```python
from build123d import *

# Parameters (mm, degrees)
SKETCH_1_R               = 22.5
EXTRUDE_1_DEPTH          = 9.5
SKETCH_2_R               = 15
EXTRUDE_2_DEPTH          = 5
SKETCH_3_R               = 1.5
CUT_EXTRUDE_1_DEPTH      = 5
SKETCH_5_R               = 1.5
CUT_EXTRUDE_2_DEPTH      = 34.207679835
CUT_EXTRUDE_6_DEPTH      = 3
PATTERN_CIRCULAR_1_COUNT = 12


with BuildPart() as part:
    # 草图1 → 凸台-拉伸1 (new body)
    with BuildSketch(Plane.XY):
        Circle(SKETCH_1_R)
    extrude(amount=EXTRUDE_1_DEPTH)

    # 草图2 → 凸台-拉伸2 (add)
    with BuildSketch(Plane.XY.offset(9.5)):
        Circle(SKETCH_2_R)
    extrude(amount=EXTRUDE_2_DEPTH)

    # 草图3 → 切除-拉伸1 (cut)
    with BuildSketch(Plane.XY.offset(9.5)):
        with Locations((0, 18.5)):
            Circle(SKETCH_3_R)
    cut_extrude_1 = extrude(amount=-CUT_EXTRUDE_1_DEPTH, mode=Mode.SUBTRACT)

    # 草图5 → 切除-拉伸2 (cut, through all)
    with BuildSketch(Plane.XY.offset(9.5)):
        with Locations((0, 18.5)):
            Circle(SKETCH_5_R)
    cut_extrude_2 = extrude(amount=-CUT_EXTRUDE_2_DEPTH, mode=Mode.SUBTRACT)

    # 草图9 → 切除-拉伸6 (cut)
    with BuildSketch(Plane(origin=(0, 0, 0), x_dir=(-1, 0, 0), z_dir=(0, 0, -1))):
        Polygon((1.204492644, 21.438116881), (-1.942237536, 21.012179669), (-3.14673018, 18.074062788), (-1.204492644, 15.561883119), (1.942237536, 15.987820331), (3.14673018, 18.925937212), align=None)
    cut_extrude_6 = extrude(amount=-CUT_EXTRUDE_6_DEPTH, mode=Mode.SUBTRACT)

    # 阵列(圆周)1: 切除-拉伸1, 切除-拉伸2, 切除-拉伸6 ×12 about axis
    pattern_circular_1_axis = Axis((0, 0, 0), (0, 0, 1))
    add([cut_extrude_1.rotate(pattern_circular_1_axis, i * 360 / PATTERN_CIRCULAR_1_COUNT) for i in range(1, PATTERN_CIRCULAR_1_COUNT)], mode=Mode.SUBTRACT)
    add([cut_extrude_2.rotate(pattern_circular_1_axis, i * 360 / PATTERN_CIRCULAR_1_COUNT) for i in range(1, PATTERN_CIRCULAR_1_COUNT)], mode=Mode.SUBTRACT)
    add([cut_extrude_6.rotate(pattern_circular_1_axis, i * 360 / PATTERN_CIRCULAR_1_COUNT) for i in range(1, PATTERN_CIRCULAR_1_COUNT)], mode=Mode.SUBTRACT)


solid = part.part
```
Could you check a few things on this model? Use its own coordinates, in mm. A direction names the side the tool comes from. Give positions to 0.01 mm unless a question says otherwise; leave off trailing zeros. Order: outer loops, then holes, each group sorted by start corner. A loop starts at its lowest first (then second) coordinate and runs counter-clockwise, first axis right, second up.
Q1. Suppose I cut it at C-C, the plane z = 4.75. Count the separate pieces of the cut face and the enclosed holes in it, and give its area (3 significant figures).
Q2. Suppose I cut it at D-D, the plane y = 5.5. Write out the boundary of the cut face in (x, z).
Q3. Suppose I cut it at A-A, the plane y = 0. Write out the boundary of the cut face in (x, z), and give its area (3 significant figures).
Q4. Suppose I cut it at B-B, the plane x = 4.5. Write out the boundary of the cut face in (y, z), and give its area (3 significant figures).
Q5. We'd pull the mould along Y, two halves only. Please class faces 1 (the flat face through (8.186, -13.485, 1.479)), 2 (the cylindrical face through (10.382, -19.961, 4.684)): +Y half, -Y half, draft (parallel to the pull), parting line (faces both ways), or undercut.
Q6. If I drill on line 1 along Y through (x, z) = (0, 7.75); line 2 along X through (y, z) = (16, 8.25); line 3 along Z through (x, y) = (-17, -14), over which ranges is the centre line in solid material (lowest first)?
Q7. I'm going to push flat-ended pins straight in: P1, Ø2.5, axis at x = 18.5, y = 0, coming from the +Z side; P2, Ø3, axis at x = 16, y = 10, coming from the -Z side; P3, Ø1, axis at x = 3, z = 1.5, coming from the +Y side; P4, Ø5, axis at x = -16.02, y = -9.25, coming from the +Z side. Where does each tip first touch, or does it pass through?
Q8. For faces 3 (the flat face through (-16.836, 2.189, 1.479)), 4 (the cylindrical face through (9.825, -14.636, 6.296)), which set-ups out of +Z, -Z, +X, -X, +Y, -Y let a thin tool reach every point of the face, with its end or its side?
Solution:
1. separate pieces: 1
1. enclosed holes: 12
1. area: 1,510 mm2
2. outline: (-21.82, 0) - (21.82, 0) - (21.82, 9.5) - (13.96, 9.5) - (13.96, 14.5) - (-13.96, 14.5) - (-13.96, 9.5) - (-21.82, 9.5) - close
3. outline: (-22.5, 0) - (-21.28, 0) - (-21.28, 3) - (-20, 3) - (-20, 9.5) - (-22.5, 9.5) - close; (-17, 3) - (-15.72, 3) - (-15.72, 0) - (15.72, 0) - (15.72, 3) - (17, 3) - (17, 9.5) - (15, 9.5) - (15, 14.5) - (-15, 14.5) - (-15, 9.5) - (-17, 9.5) - close; (20, 3) - (21.28, 3) - (21.28, 0) - (22.5, 0) - (22.5, 9.5) - (20, 9.5) - close
3. area: 505 mm2
4. outline: (-22.05, 0) - (22.05, 0) - (22.05, 9.5) - (14.31, 9.5) - (14.31, 14.5) - (-14.31, 14.5) - (-14.31, 9.5) - (-22.05, 9.5) - close
4. area: 562 mm2
5. face 1: undercut
5. face 2: parting line
6. line 1: y = -22.5 to -20, -17 to 17, 20 to 22.5
6. line 2: x = -15.82 to -10.75, -7.75 to 7.75, 10.75 to 15.82
6. line 3: z = 0 to 9.5
7. P1: passes through
7. P2: stops at z = 3
7. P3: stops at y = 22.36
7. P4: stops at z = 9.5
8. face 3: -Z
8. face 4: +Z, -Z
